```python
from build123d import *

# Parameters (mm, degrees)
CROQUIS1_W              = 10
CROQUIS1_H              = 27
SALIENTE_EXTRUIR1_DEPTH = 2.6
CROQUIS2_W              = 10
CROQUIS2_H              = 4
SALIENTE_EXTRUIR2_DEPTH = 6.2
CROQUIS3_W              = 10
CROQUIS3_H              = 1.5
SALIENTE_EXTRUIR3_DEPTH = 6
CROQUIS4_R              = 1.55
CORTAR_EXTRUIR1_DEPTH   = 5
SIMETR_A1_START         = 2.6
SIMETR_A1_OUTLINE_W     = 10
SIMETR_A1_OUTLINE_H     = 4
SIMETR_A1_DEPTH         = 6.2
SIMETR_A1_START_2       = 7.3
SIMETR_A1_2_OUTLINE_W   = 10
SIMETR_A1_2_OUTLINE_H   = 6
SIMETR_A1_2_OUTLINE_R   = 1.55
SIMETR_A1_2_DEPTH       = 1.5


# Read off the part's stored shape, not the designer's step: Simetr_a1
with BuildPart() as part:
    # Croquis1 → Saliente-Extruir1 (new body)
    with BuildSketch(Plane(origin=(0, 0, 0), x_dir=(1, 0, 0), z_dir=(0, 1, 0))):
        Rectangle(CROQUIS1_W, CROQUIS1_H)
    extrude(amount=SALIENTE_EXTRUIR1_DEPTH)

    # Croquis2 → Saliente-Extruir2 (add)
    with BuildSketch(Plane(origin=(0, 2.6, 0), x_dir=(1, 0, 0), z_dir=(0, 1, 0))):
        with Locations((0, 11.5)):
            Rectangle(CROQUIS2_W, CROQUIS2_H)
    extrude(amount=SALIENTE_EXTRUIR2_DEPTH)

    # Croquis3 → Saliente-Extruir3 (add)
    with BuildSketch(Plane(origin=(0, 0, -13.5), x_dir=(-1, 0, 0), z_dir=(0, 0, -1))):
        with Locations((0, 8.05)):
            Rectangle(CROQUIS3_W, CROQUIS3_H)
    extrude(amount=SALIENTE_EXTRUIR3_DEPTH)

    # Croquis4 → Cortar-Extruir1 (cut)
    with BuildSketch(Plane.XZ.offset(-7.3)):
        with Locations((0, -16.5)):
            Circle(CROQUIS4_R)
    extrude(amount=-CORTAR_EXTRUIR1_DEPTH, mode=Mode.SUBTRACT)

    # Simetr_a1 outline → Simetr_a1 (add)
    with BuildSketch(Plane(origin=(0, 0, 0), x_dir=(1, 0, 0), z_dir=(0, 1, 0)).offset(SIMETR_A1_START)):
        with Locations((0, -11.5)):
            Rectangle(SIMETR_A1_OUTLINE_W, SIMETR_A1_OUTLINE_H)
    extrude(amount=SIMETR_A1_DEPTH)

    # Simetr_a1 2 outline → Simetr_a1 2 (add)
    with BuildSketch(Plane(origin=(0, 0, 0), x_dir=(1, 0, 0), z_dir=(0, 1, 0)).offset(SIMETR_A1_START_2)):
        with Locations((0, -16.5)):
            Rectangle(SIMETR_A1_2_OUTLINE_W, SIMETR_A1_2_OUTLINE_H)
        with Locations((0, -16.5)):
            Circle(SIMETR_A1_2_OUTLINE_R, mode=Mode.SUBTRACT)
    extrude(amount=SIMETR_A1_2_DEPTH)


solid = part.part
```
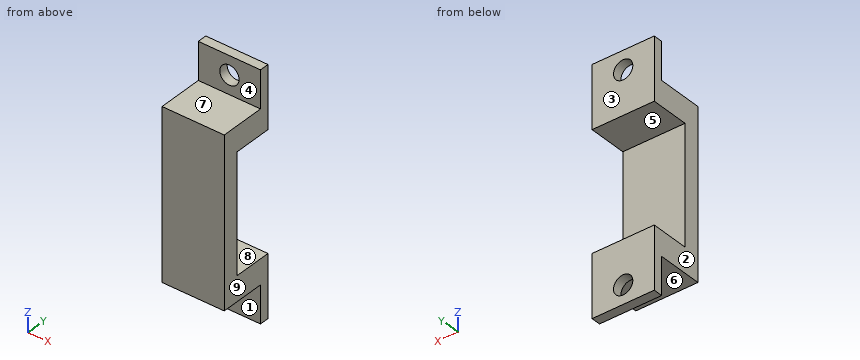
Input: part model. Units: mm. Frame: model coordinates. Face numbers are marked on the shaded views. A direction names the side the tool comes from. Coordinates: 2 decimals unless noted, no trailing zeros. Order: outer loops, then holes, each group sorted by start corner. A loop starts at its lowest first (then second) coordinate and runs counter-clockwise, first axis right, second up. Notation, with made-up numbers: (-8.5, 15) - (47.5, 15) arc R21 cw to (47.5, 35) - close; hole circle Ø4 at (74, -6.5). An arc over 180 degrees is marked (long way). Return JSON: item names as keys, results as strings.
Q1. Cut plane B-B (y = 3). Return loops of the section in (x, z), then the cut area to 3 significant figures.
The answers:
{"outline": "(-5, -13.5) - (5, -13.5) - (5, -9.5) - (-5, -9.5) - close; (-5, 9.5) - (5, 9.5) - (5, 13.5) - (-5, 13.5) - close", "area": "80.0 mm2"}
Q2. Ray query, probe 1 along Z at (x, y) = (0, 8.4); probe 2 along Z at (x, y) = (-1.75, 4.5); probe 3 along X at (y, z) = (8.05, 16.5). Return the intervals inside material, ascending.
The answers:
{"probe 1": "z = -19.5 to -18.05, -14.95 to -9.5, 9.5 to 14.95, 18.05 to 19.5", "probe 2": "z = -13.5 to -9.5, 9.5 to 13.5", "probe 3": "x = -5 to -1.55, 1.55 to 5"}
Q3. Draft query along Z for the marked faces 6, 7, 8 and 9. Return one class per face: +Z half, -Z half, draft (parallel to the pull), parting line (faces both ways), or undercut.
The answers:
{"face 6": "-Z half", "face 7": "+Z half", "face 8": "undercut", "face 9": "draft"}
Q4. First-contact query: pin 1 (3 mm diameter, centred on x = 0, y = 5.5, fed in from +Z); pin 2 (3 mm diameter, centred on x = 0, z = 16.5, fed in from -Y); pin 3 (2 mm diameter, centred on x = 3, z = -3.5, fed in from +Y); pin 4 (3 mm diameter, centred on x = -2, z = 18, fed in from -Y). Flat tips, straight axial feed; report the tip coordinate or a pass-through.
The answers:
{"pin 1": "stops at z = 13.5", "pin 2": "passes through", "pin 3": "stops at y = 2.6", "pin 4": "stops at y = 7.3"}
Q5. Cut plane D-D (x = -3). Return loops of the section in (y, z), then the cut area to 3 significant figures.
The answers:
{"outline": "(0, -13.5) - (7.3, -13.5) - (7.3, -19.5) - (8.8, -19.5) - (8.8, -9.5) - (2.6, -9.5) - (2.6, 9.5) - (8.8, 9.5) - (8.8, 19.5) - (7.3, 19.5) - (7.3, 13.5) - (0, 13.5) - close", "area": "138 mm2"}
Q6. Cut plane A-A (z = -16.5). Return loops of the section in (x, y), then the cut area to 4 significant figures.
The answers:
{"outline": "(-5, 7.3) - (-1.55, 7.3) - (-1.55, 8.8) - (-5, 8.8) - close; (1.55, 7.3) - (5, 7.3) - (5, 8.8) - (1.55, 8.8) - close", "area": "10.35 mm2"}
Q7. Cut plane C-C (x = 0). Return loops of the section in (y, z).
The answers:
{"outline": "(0, -13.5) - (7.3, -13.5) - (7.3, -14.95) - (8.8, -14.95) - (8.8, -9.5) - (2.6, -9.5) - (2.6, 9.5) - (8.8, 9.5) - (8.8, 14.95) - (7.3, 14.95) - (7.3, 13.5) - (0, 13.5) - close; (7.3, -19.5) - (8.8, -19.5) - (8.8, -18.05) - (7.3, -18.05) - close; (7.3, 18.05) - (8.8, 18.05) - (8.8, 19.5) - (7.3, 19.5) - close"}
Q8. Access query for the marked faces 1, 2, 3, 4 and 5. Directions: +Z, -Z, +X, -X, +Y, -Y. A direction counts if a zero-diameter tool reaches every point of the face in a straight line with its end or side. Return the directions, or none.
The answers:
{"face 1": "-Z, +X, -X, -Y", "face 2": "+Z, -Z, -X, +Y, -Y", "face 3": "+Z, -Z, +X, -X, +Y", "face 4": "+Z, +X, -X, -Y", "face 5": "+X, -X, +Y"}
